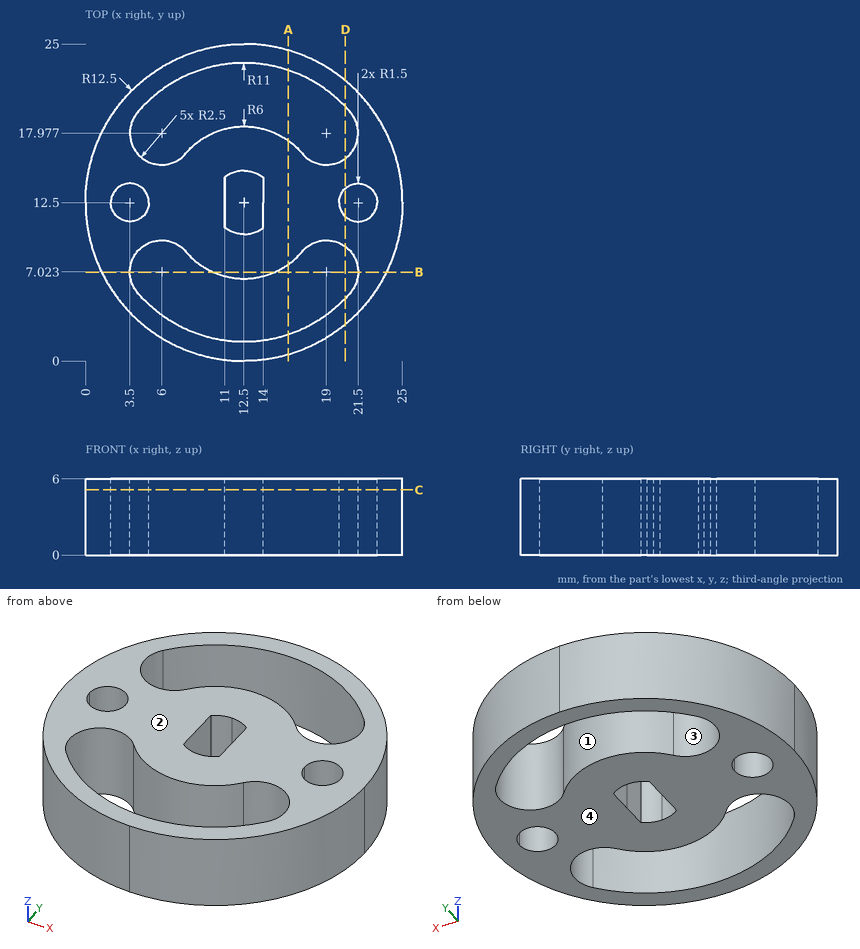
Print and shaded views of the part. All mm, measured from the part's lowest x, y and z. A direction names the side the tool comes from. Round coordinates to 2 decimals unless told otherwise and drop trailing zeros. Write each loop counter-clockwise with the first axis right and the second up, starting at its lowest first coordinate (ties: lowest second). Pieces come first, ordered by that corner, then holes. Notation, with made-up numbers: (77, 65.5) -> (92, 65.5) arc R18 cw to (92, 95.5) -> close; hole circle Ø1 at (-37, 30). An arc over 180 degrees is marked (long way). Answer in a Markdown table with one row per item. Add a question column.
Item 1: Drop flat-ended pins along their axis: pin 1 Ø12 at (x, y) = (11.5, 9.5) entering from -Z; pin 2 Ø2 at (y, z) = (4, 3) entering from -X; pin 3 Ø1.5 at (y, z) = (9.5, 4) entering from +X. Give the stop position or say it passes through.
Item 2: Saw through at D-D, the plane x = 20.5. Count the separate pieces of the cut face and the enclosed holes in it.
Item 3: Drill centre lines: line 1 (Y direction, x = 16.25, z = 0.9) (1 decimal); line 2 (Y direction, x = 6.5, z = 4.85) (1 decimal); line 3 (Y direction, x = 4.75, z = 4.55) (1 decimal). Where is each one in solid material? Low to high. Write a range as from..to.
Item 4: Saw through at A-A, the plane x = 16. Write the cut outline in (y, z).
Item 5: Which spindle directions (+Z, -Z, +X, -X, +Y, -Y) get a long thin tool onto all of the face, cutting with end or side? Do the marked faces 1 and 2. Say none if no direction does.
Item 6: Saw through at C-C, the plane z = 5.15. Write the cut outline in (x, y).
Item 7: Mould opens along X. For the marked faces 3 and 4 say: pulls with the +X half, pulls with the -X half, needs draft (parallel to the pull), parting line crosses it, or undercut.
Item 8: Saw through at B-B, the plane y = 7. Write the cut outline in (x, z) (1 decimal).
Findings below:
| question | item | result |
|---|---|---|
| 1 | pin 1 | stops at z = 0 |
| 1 | pin 2 | stops at x = 2.5 |
| 1 | pin 3 | stops at x = 24.8 |
| 2 | separate pieces | 4 |
| 2 | enclosed holes | 0 |
| 3 | line 1 | y = 0.6..2.2, 7.8..17.2, 22.8..24.4 |
| 3 | line 2 | y = 1.5..3.3, 9.5..15.5, 21.7..23.5 |
| 3 | line 3 | y = 2.7..4.7, 9.2..11.7, 13.3..15.8, 20.3..22.3 |
| 4 | outline | (0.5, 0) -> (2.07, 0) -> (2.07, 6) -> (0.5, 6) -> close; (7.63, 0) -> (17.37, 0) -> (17.37, 6) -> (7.63, 6) -> close; (22.93, 0) -> (24.5, 0) -> (24.5, 6) -> (22.93, 6) -> close |
| 5 | face 1 | +Z, -Z |
| 5 | face 2 | +Z, +X, -X, +Y, -Y |
| 6 | outline | circle Ø25 at (12.5, 12.5); hole circle Ø3 at (3.5, 12.5); hole (4.09, 5.41) arc R11 ccw to (20.91, 5.41) arc R2.5 ccw to (17.09, 8.63) arc R6 cw to (7.91, 8.63) arc R2.5 ccw to start; hole (4.09, 19.59) arc R2.5 ccw to (7.91, 16.37) arc R6 cw to (17.09, 16.37) arc R2.5 ccw to (20.91, 19.59) arc R11 ccw to start; hole (11, 10.5) arc R2.5 ccw to (14, 10.5) -> (14, 14.5) arc R2.5 ccw to (11, 14.5) -> close; hole circle Ø3 at (21.5, 12.5) |
| 7 | face 3 | undercut |
| 7 | face 4 | needs draft |
| 8 | outline | (1.3, 0) -> (3.5, 0) -> (3.5, 6) -> (1.3, 6) -> close; (10.1, 0) -> (14.9, 0) -> (14.9, 6) -> (10.1, 6) -> close; (21.5, 0) -> (23.7, 0) -> (23.7, 6) -> (21.5, 6) -> close |
